Can you work these out from the model? Positions are in its coordinate system, mm. Face numbers are marked on the shaded views. Give positions to 0.01 mm unless a question says otherwise; leave off trailing zeros. Loops run counter-clockwise (first coordinate to the right, second up) from the corner with the lowest first, then second, coordinate; pieces in that order, holes last.
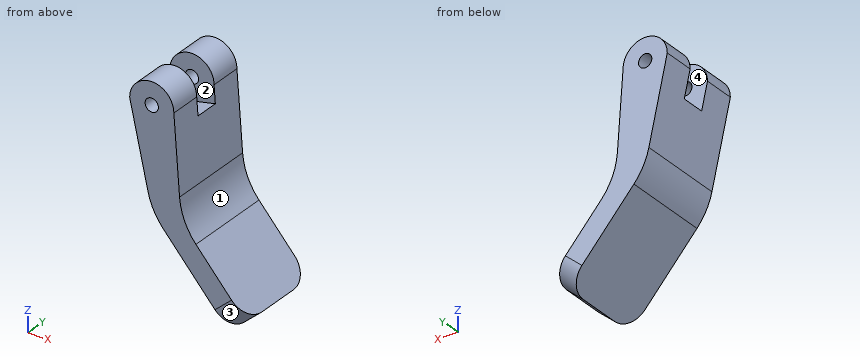
from build123d import *

# Parameters (mm, degrees)
BOSS_EXTRUDE1_DEPTH = 40
FILLET1_R           = 10
FILLET2_R           = 30
FILLET3_R           = 30
SKETCH3_R           = 3
CUT_EXTRUDE1_DEPTH  = 50
SKETCH5_W           = 20
SKETCH5_H           = 11
CUT_EXTRUDE2_DEPTH  = 50


with BuildPart() as part:
    # Sketch2 → Boss-Extrude1 (new body)
    with BuildSketch(Plane(origin=(0, 0, 0), x_dir=(1, 0, 0), z_dir=(0, 1, 0))):
        with BuildLine():
            Line((-10, 0), (0, 45))
            Line((0, 45), (35.22081686, 85))
            Line((35.22081686, 85), (42.726014623, 78.391520103))
            Line((42.726014623, 78.391520103), (13.324099267, 45))
            Line((13.324099267, 45), (10, 0))
            ThreePointArc((10, 0), (0, -10), (-10, 0))
        make_face()
    extrude(amount=BOSS_EXTRUDE1_DEPTH)

    # Fillet1
    fillet1_edges = [part.edges().sort_by_distance(p)[0] for p in [
        (38.973415741, 40, -81.695760051),
        (38.973415741, 0, -81.695760051),
    ]]
    fillet(fillet1_edges, radius=FILLET1_R)

    # Fillet2
    fillet2_edges = [part.edges().sort_by_distance(p)[0] for p in [
        (0, 20, -45),
    ]]
    fillet(fillet2_edges, radius=FILLET2_R)

    # Fillet3
    fillet3_edges = [part.edges().sort_by_distance(p)[0] for p in [
        (13.324099267, 20, -45),
    ]]
    fillet(fillet3_edges, radius=FILLET3_R)

    # Sketch3 → Cut-Extrude1 (cut)
    with BuildSketch(Plane(origin=(0, 40, 0), x_dir=(1, 0, 0), z_dir=(0, 1, 0))):
        with Locations(Location((0, 0, 0), (0, 0, 270))):
            Circle(SKETCH3_R)
    extrude(amount=-CUT_EXTRUDE1_DEPTH, mode=Mode.SUBTRACT)

    # Sketch5 → Cut-Extrude2 (cut)
    with BuildSketch(Plane(origin=(-9.529411765, 0, -2.117647059), x_dir=(-0.21693045781865625, 0, 0.9761870601839528), z_dir=(-0.9761870601839528, 0, -0.21693045781865625))):
        with Locations((0, 20)):
            Rectangle(SKETCH5_W, SKETCH5_H)
    extrude(amount=-CUT_EXTRUDE2_DEPTH, mode=Mode.SUBTRACT)


solid = part.part
(1) Thinking about a two-plate mould opening in Y: for the marked faces 1, 2, 3 and 4, which applies, pulls with the +Y half, pulls with the -Y half, needs draft (parallel to the pull), parting line crosses it, or undercut?
Returned:
face 1: needs draft
face 2: undercut
face 3: pulls with the -Y half
face 4: undercut
(2) Suppose I cut it at A-A on y = 16. List the corners of the cut face in (x, z) for me.
Returned:
outline: (-7.36, -11.88) - (-1.67, -37.47) arc R30 ccw to (5.1, -50.79) - (35.22, -85) - (42.73, -78.39) - (19.98, -52.56) arc R30 cw to (12.58, -34.95) - (10.58, -7.89) - close
(3) Suppose I cut it at D-D on y = 32. List the corners of the cut face in (x, z) for me.
Returned:
outline: (-10, 0) - (-1.67, -37.47) arc R30 ccw to (5.1, -50.79) - (35.09, -84.85) - (42.59, -78.24) - (19.98, -52.56) arc R30 cw to (12.58, -34.95) - (10, 0) arc R10 ccw to start; hole circle Ø6 at (0, 0)
(4) Suppose I cut it at B-B on x = 0. List the corners of the cut face in (y, z) for me, plus the area to 3 significant figures.
Returned:
outline: (0, -42.69) - (40, -42.69) - (40, -3) - (25.5, -3) - (25.5, -10.24) - (14.5, -10.24) - (14.5, -3) - (0, -3) - close; (0, 3) - (14.5, 3) - (14.5, 10) - (0, 10) - close; (25.5, 3) - (40, 3) - (40, 10) - (25.5, 10) - close
area: 1,710 mm2
(5) Will these pins go through, and if not, where does the flat tip stop? P1, Ø6, axis at y = 23.5, z = -58.5, coming from the +X side; P2, Ø3.5, axis at x = 0, z = 0, coming from the -Y side; P3, Ø1, axis at x = 18.5, y = 22, coming from the +Z side; P4, Ø6, axis at x = -1.5, z = -2, coming from the +Y side.
Returned:
P1: stops at x = 27.85
P2: passes through
P3: stops at z = -50.05
P4: stops at y = 40
(6) Please list where these lines run through material, in increasing order: probe 1 along X at (y, z) = (7, 0); probe 2 along Z at (x, y) = (1.5, 35); probe 3 along X at (y, z) = (5, 1).
Returned:
probe 1: x = -10 to -3, 3 to 10
probe 2: z = -45.73 to -2.6, 2.6 to 9.89
probe 3: x = -9.95 to -2.83, 2.83 to 9.95
(7) Suppose I cut it at C-C on x = 8.5. List the corners of the cut face in (y, z) for me.
Returned:
outline: (0, -54.65) - (40, -54.65) - (40, 5.27) - (25.5, 5.27) - (25.5, -8.36) - (14.5, -8.36) - (14.5, 5.27) - (0, 5.27) - close
